```python
from build123d import *

# Parameters (mm, degrees)
F0_R     = 21.844
F1_DEPTH = 2.54
F2_R     = 21.844
F2_R_2   = 19.304
F3_R     = 15.621
F3_R_2   = 13.081
F4_DEPTH = 5.08


with BuildPart() as f1:
    # F0 (on Top) → F1 (new body)
    with BuildSketch(Plane.XY):
        Circle(F0_R)
    extrude(amount=F1_DEPTH)

    # F2 (on face) + F3 (on face) → F4 (join)
    with BuildSketch(Plane.XY.offset(2.54)):
        Circle(F2_R)
        Circle(F2_R_2, mode=Mode.SUBTRACT)
    with BuildSketch(Plane.XY.offset(2.54)):
        Circle(F3_R)
        Circle(F3_R_2, mode=Mode.SUBTRACT)
    extrude(amount=F4_DEPTH)


solid = f1.part
```
Geometry: final body of the model. Coordinates: model frame, mm. A direction names the side the tool comes from. Round coordinates to 2 decimals unless told otherwise and drop trailing zeros. Loops run counter-clockwise (first coordinate to the right, second up) from the corner with the lowest first, then second, coordinate; pieces in that order, holes last.
Item 1: Line query: L1, parallel to Y at x = 0, z = 4; L2, parallel to Y at x = -9.5, z = 5; L3, parallel to X at y = 2, z = 6. Output: solid intervals per line, ascending.
Checked values:
L1: y = -21.84 to -19.3, -15.62 to -13.08, 13.08 to 15.62, 19.3 to 21.84
L2: y = -19.67 to -16.8, -12.4 to -8.99, 8.99 to 12.4, 16.8 to 19.67
L3: x = -21.75 to -19.2, -15.49 to -12.93, 12.93 to 15.49, 19.2 to 21.75
Item 2: Reachability of faces 1 (the cylindrical face through (-1.7, 12.97, 5.04)), 2 (the flat face through (-4, -13, 7.62)) from +Z, -Z, +X, -X, +Y, -Y: full face, straight path, thin tool, end or side. Return the list, or none.
Checked values:
face 1: +Z
face 2: +Z, +X, -X, +Y, -Y
Item 3: Mould query, pull axis X, two halves, no side actions, for faces 3 (the flat face through (8, -18, 7.62)), 4 (the cylindrical face through (20.835, 6.561, 3.757)), 5 (the cylindrical face through (-15.319, -11.746, 5.044)). Classes: released by +X, released by -X, zero draft, split by the parting line, or undercut.
Checked values:
face 3: zero draft
face 4: split by the parting line
face 5: undercut
Item 4: Section D-D, the plane y = -18.5. Output: boundary loops of the cut face in (x, z), plus the area to 3 significant figures.
Checked values:
outline: (-11.62, 0) - (11.62, 0) - (11.62, 7.62) - (5.51, 7.62) - (5.51, 2.54) - (-5.51, 2.54) - (-5.51, 7.62) - (-11.62, 7.62) - close
area: 121 mm2
Item 5: Contact query for flat-ended pins moving along their axis: P1, Ø5, axis at x = 7, y = 0.5, coming from the +Z side; P2, Ø3, axis at x = 4, z = 4, coming from the -Y side; P3, Ø4, axis at y = -11.5, z = 1.5, coming from the -X side. Output: stop coordinate, or through.
Checked values:
P1: stops at z = 2.54
P2: stops at y = -21.7
P3: stops at x = -19.67
Item 6: Section B-B, the plane y = 0. Output: boundary loops of the cut face in (x, z).
Checked values:
outline: (-21.84, 0) - (21.84, 0) - (21.84, 7.62) - (19.3, 7.62) - (19.3, 2.54) - (15.62, 2.54) - (15.62, 7.62) - (13.08, 7.62) - (13.08, 2.54) - (-13.08, 2.54) - (-13.08, 7.62) - (-15.62, 7.62) - (-15.62, 2.54) - (-19.3, 2.54) - (-19.3, 7.62) - (-21.84, 7.62) - close
Item 7: Section A-A, the plane z = 6.25. Output: boundary loops of the cut face in (x, y).
Checked values:
outline: circle Ø43.69 at (0, 0); circle Ø31.24 at (0, 0); hole circle Ø38.61 at (0, 0); hole circle Ø26.16 at (0, 0)
